The listing builds one solid part. Answer for the finished solid, in the listing's coordinates (mm). Face numbers are marked on the shaded views. A direction names the side the tool comes from. Coordinates: 2 decimals unless noted, no trailing zeros. Loops run counter-clockwise (first coordinate to the right, second up) from the corner with the lowest first, then second, coordinate; pieces in that order, holes last. Notation, with made-up numbers: M 83.5,81 L 106.5,81 A34 cw 106.5,119 Z; hole C 59.25,-10 d9. An arc over 180 degrees is marked long. Return JSON: item names as keys, results as strings. Group by question number.
1. Section A-A (y = 55) is taken. Write down the section's boundary in (x, z), then the cut area to 3 significant figures.
2. Which of the six approach directions +Z, -Z, +X, -X, +Y, -Y give full straight-line access (tool end or side, diameter ignored) to the marked faces 1, 2 and 3?
3. Given P1, Ø8.5, axis at x = 11, y = 81.5, coming from the +Z side; P2, Ø8, axis at x = 11, z = 6, coming from the -Y side; P3, Ø4, axis at x = 10.5, z = 11.5, coming from the +Y side; P4, Ø10, axis at x = 18.5, z = 17, coming from the -Y side, each flat-ended and moving along its own axis, determine where each tip first touches the part or whether it passes through.
4. Straight lines are drawn through the part: L1, parallel to Y at x = 23.75, z = 8; L2, parallel to X at y = 34.7, z = 13; L3, parallel to Y at x = 12.25, z = 20. For each, find the intervals that lie inside material, in ascending order. Write a range as from..to.
5. Section C-C (z = 8) is taken. Write down the section's boundary in (x, y).
6. Section D-D (z = 20) is taken. Write down the section's boundary in (x, y).
7. Section B-B (x = 18.95) is taken. Count the separate pieces of the cut face and the enclosed holes in it, then the cut area to 3 significant figures.
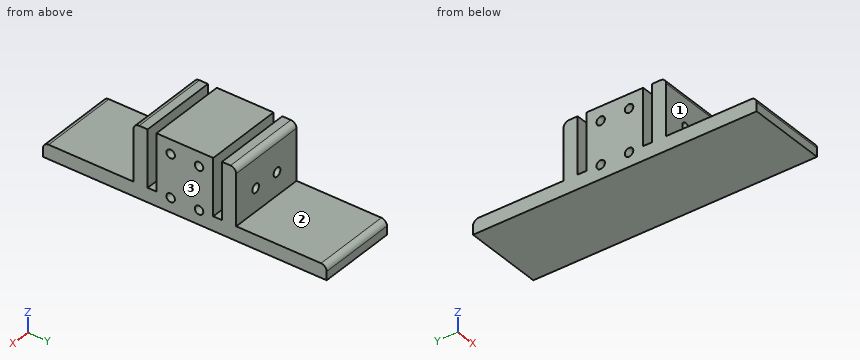
Autodesk Inventor part; units mm, degrees
ref_plane "YZ Plane" through (0, 0, 0) normal (1, 0, 0) x (0, 1, 0)
ref_plane "XZ Plane" through (0, 0, 0) normal (0, 1, 0) x (-1, 0, 0)
ref_plane "XY Plane" through (0, 0, 0) normal (0, 0, 1) x (1, 0, 0)
sketch "Sketch1" plane through (0, 0, 0) normal (0, 0, 1) x (1, 0, 0)
  line L0 (0, 0) -> (28, 0)
  line L1 (28, 0) -> (28, 100)
  line L2 (28, 100) -> (0, 100)
  line L3 (0, 100) -> (0, 0)
  dimension "d0" = 28
  dimension "d1" = 100
extrude "Extrusion1" add sketch "Sketch1" along normal blind 5
sketch "Sketch3" plane through (0, 0, 5) normal (0, 0, 1) x (1, 0, 0)
  line L0 (28, 0) -> (28, 100)
  line L1 (28, 100) -> (0, 100)
  line L2 (0, 100) -> (0, 0)
  line L3 (0, 0) -> (28, 0)
  line L4 (0, 50) -> (28, 50) construction
  line L5 (28, 0) -> (28, 100) construction
  line L6 (0, 100) -> (0, 0)
  line L7 (0, 60) -> (28, 60)
  line L8 (28, 60) -> (28, 40)
  line L9 (28, 40) -> (0, 40)
  line L10 (0, 40) -> (0, 60)
  line L11 (0, 63.1) -> (28, 63.1)
  line L12 (28, 63.1) -> (28, 68.1)
  line L13 (28, 68.1) -> (0, 68.1)
  line L14 (0, 68.1) -> (0, 63.1)
  line L15 (0, 36.9) -> (28, 36.9)
  line L16 (28, 36.9) -> (28, 31.9)
  line L17 (28, 31.9) -> (0, 31.9)
  line L18 (0, 31.9) -> (0, 36.9)
  point P0 (0, 31.9)
  point P1 (28, 36.9)
  point P2 (0, 40)
  point P3 (0, 68.1)
  point P4 (28, 63.1)
  dimension "d6" = 50
  dimension "d7" = 100
  dimension "d8" = 10
  dimension "d9" = 10
  dimension "d10" = 5
  dimension "d11" = 3.1
  dimension "d12" = 3.1
  dimension "d13" = 5
extrude "Extrusion2" add sketch "Sketch3" along normal blind 20 contours L17 L2 L15 L0 | L9 L2 L7 L0 | L11 L2 L13 L0
sketch "Sketch4" plane through (0, 68.1, 5) normal (0, 1, 0) x (1, 0, 0)
  line L0 (0, 0) -> (28, 0)
  line L1 (0, 0) -> (0, -20)
  line L2 (28, -20) -> (0, -20)
  line L3 (28, 0) -> (28, -20)
  circle A0 centre (9.05, -8) radius 1.55
  circle A1 centre (18.95, -8) radius 1.55
  line L4 (0, -20) -> (28, -20) construction
  line L5 (14, -20) -> (14, 0) construction
  point P0 (0, 5)
  dimension "d16" = 3.1
  dimension "d17" = 3.1
  dimension "d18" = 4.95
  dimension "d19" = 4.95
  dimension "d20" = 8
  dimension "d21" = 8
extrude "Extrusion3" cut sketch "Sketch4" against normal blind 100 contours A0 | A1
ref_plane "Work Plane1" through (14, 0, 0) normal (1, 0, 0) x (0, 0, -1)
sketch "Sketch13" plane through (28, 0, 0) normal (1, 0, 0) x (0, 0, -1)
  circle A0 centre (-5, 55) radius 1.5
  circle A1 centre (-5, 45) radius 1.5
  circle A2 centre (-20, 55) radius 1.5
  circle A3 centre (-20, 45) radius 1.5
  line L0 (-5, 60) -> (-25, 60)
  line L1 (-5, 40) -> (-25, 40)
  line L2 (-25, 40) -> (-25, 60)
  line L3 (0, 0) -> (0, 100)
  dimension "d57" = 3
  dimension "d58" = 3
  dimension "d59" = 3
  dimension "d60" = 3
  dimension "d61" = 5
  dimension "d62" = 5
  dimension "d63" = 5
  dimension "d64" = 5
  dimension "d65" = 5
  dimension "d67" = 5
  dimension "d69" = 5
  dimension "d70" = 5
extrude "Extrusion11" cut sketch "Sketch13" against normal blind 180
fillet "Fillet1" radius 2 4 edges at (14, 100, 5) (14, 0, 5) (14, 68.1, 25) (14, 31.9, 25)
ref_plane "Work Plane3" through (0, 50, 5) normal (0, 1, 0) x (1, 0, 0)
equation "\"d6\" = 0.5 * d7"
equation "\"d62\" = d61"
equation "\"d63\" = d61"
equation "\"d64\" = d61"
equation "\"d67\" = d65"
equation "\"d69\" = d65"
equation "\"d70\" = d65"
properties part number "Foam_wing_mount"
Worked out:
{
 "1": {"outline": "M 0,0 L 28,0 L 28,3.5 L 0,3.5 Z; M 0,6.5 L 28,6.5 L 28,18.5 L 0,18.5 Z; M 0,21.5 L 28,21.5 L 28,25 L 0,25 Z; hole C 9.05,13 d3.1; hole C 18.95,13 d3.1", "area": "517 mm^2"},
 "2": {"face 1": "+Z, +X, -X, -Y", "face 2": "+Z, +X, -X, +Y", "face 3": "+Z, -Z, +X, +Y, -Y"},
 "3": {"P1": "z = 5", "P2": "y = 0", "P3": "y = 68.1", "P4": "y = 31.9"},
 "4": {"L1": "31.9..36.9, 40..60, 63.1..68.1", "L2": "0..7.5, 10.6..17.4, 20.5..28", "L3": "31.9..36.9, 40..43.5, 46.5..53.5, 56.5..60, 63.1..68.1"},
 "5": {"outline": "M 0,31.9 L 28,31.9 L 28,36.9 L 0,36.9 Z; M 0,40 L 28,40 L 28,60 L 0,60 Z; M 0,63.1 L 28,63.1 L 28,68.1 L 0,68.1 Z"},
 "6": {"outline": "M 0,31.9 L 28,31.9 L 28,36.9 L 0,36.9 Z; M 0,40 L 28,40 L 28,43.5 L 0,43.5 Z; M 0,46.5 L 28,46.5 L 28,53.5 L 0,53.5 Z; M 0,56.5 L 28,56.5 L 28,60 L 0,60 Z; M 0,63.1 L 28,63.1 L 28,68.1 L 0,68.1 Z"},
 "7": {"separate pieces": "4", "enclosed holes": "4", "area": "975 mm^2"}
}
